For this review, take the finished solid that the model builds, in its own axes (mm). A direction names the side the tool comes from. Coordinates: 2 decimals unless noted, no trailing zeros.
1. Clearance check with flat-ended pins moving along their axes: P1, Ø7, axis at x = -2.5, y = 6, coming from the -Z side; P2, Ø2, axis at x = 0.5, y = 0, coming from the -Z side; P3, Ø3, axis at x = -0.5, y = -4.5, coming from the +Z side; P4, Ø5, axis at x = -2, z = 30, coming from the -Y side. State where each tip first meets the part, or that it passes through.
2. Mouldability with a two-part tool opening along X and no side actions: class faces 4 (the face through (-9, 3.5, 21)), 5 (the face through (0, 14, 18)) as pulls with the +X half, pulls with the -X half, needs draft (parallel to the pull), parting line crosses it, or undercut.
3. Take a section at A-A, the plane y = 5.5. Count the separate pieces of the cut face and the enclosed holes in it, then the cut area to 3 significant figures.
4. To check wall thickness, follow probe 1 along Z at (x, y) = (0, 9.5); probe 2 along X at (y, z) = (12.9, 25.5); probe 3 along Z at (x, y) = (-9, -6.25). State the ranges of each line that lie inside material, in increasing order.
5. Machinability: for faces 1 (the face through (0, -14, 1)), 2 (the face through (8.26, 0.39, 1.23)), 3 (the face through (0.46, 7.44, 5.81)), which of the approach directions +Z, -Z, +X, -X, +Y, -Y give a long, thin tool a straight path to every point of the face, cutting with its end or side? Answer none if there is none.
```python
from build123d import *

# Parameters (mm, degrees)
SKETCH1_W           = 33
SKETCH1_H           = 28
BOSS_EXTRUDE1_DEPTH = 46
CUT_EXTRUDE1_DEPTH  = 59.318093247
CUT_EXTRUDE2_START  = -3
CUT_EXTRUDE2_DEPTH  = 27
FILLET1_R           = 12.5
FILLET2_R           = 16.5
FILLET3_R           = 6
SKETCH4_W           = 13
SKETCH4_H           = 23
CUT_EXTRUDE3_DEPTH  = 9
SKETCH5_R           = 6.5
CUT_EXTRUDE4_DEPTH  = 56.592265809
SKETCH6_R           = 1
CUT_EXTRUDE6_DEPTH  = 8
SKETCH7_R           = 1.3
SKETCH7_R_2         = 2.5
CUT_EXTRUDE7_DEPTH  = 2.5


with BuildPart() as part:
    # Sketch1 → Boss-Extrude1 (new body)
    with BuildSketch(Plane.XY):
        Rectangle(SKETCH1_W, SKETCH1_H)
    extrude(amount=BOSS_EXTRUDE1_DEPTH)

    # Sketch2 → Cut-Extrude1 (cut, through all)
    with BuildSketch(Plane(origin=(16.5, 0, 0), x_dir=(0, 0, -1), z_dir=(1, 0, 0))):
        with BuildLine():
            Line((-46, 2), (-46, -14))
            Line((-46, -14), (-5, -14))
            add(Edge.make_bspline(
                [(-5, -14), (-24.736297584, -3.666123858), (-46, 2)],
                knots=[0, 0, 0, 1, 1, 1], degree=2))
        make_face()
    extrude(amount=-CUT_EXTRUDE1_DEPTH, mode=Mode.SUBTRACT)

    # Sketch3 → Cut-Extrude2 (cut)
    with BuildSketch(Plane(origin=(16.5, 0, 0), x_dir=(0, 0, -1), z_dir=(1, 0, 0)).offset(CUT_EXTRUDE2_START)):
        with BuildLine():
            Line((-5, -14), (-2.5, -14))
            Line((-2.5, -14), (-2.5, 3.5))
            Line((-2.5, 3.5), (-40.5, 3.5))
            Line((-40.5, 3.5), (-40.5, 0.448741524))
            add(Edge.make_bspline(
                [(-5, -14), (-22.171866916, -5.008853353), (-40.5, 0.448741524)],
                knots=[0, 0, 0, 1, 1, 1], degree=2))
        make_face()
    extrude(amount=-CUT_EXTRUDE2_DEPTH, mode=Mode.SUBTRACT)

    # Fillet1
    fillet1_edges = [part.edges().sort_by_distance(p)[0] for p in [
        (13.5, 1.974370762, 40.5),
        (-13.5, 1.974370762, 40.5),
    ]]
    fillet(fillet1_edges, radius=FILLET1_R)

    # Fillet2
    fillet2_edges = [part.edges().sort_by_distance(p)[0] for p in [
        (16.5, 8, 46),
        (-16.5, 8, 46),
    ]]
    fillet(fillet2_edges, radius=FILLET2_R - 0.0001)  # a hair under: the kernel refuses the full size

    # Fillet3
    fillet3_edges = [part.edges().sort_by_distance(p)[0] for p in [
        (-16.5, -14, 2.5),
        (16.5, -14, 2.5),
    ]]
    fillet(fillet3_edges, radius=FILLET3_R)

    # Sketch4 → Cut-Extrude3 (cut)
    with BuildSketch(Plane.XZ.offset(-3.5)):
        with Locations((0, 20.5)):
            Rectangle(SKETCH4_W, SKETCH4_H)
    extrude(amount=-CUT_EXTRUDE3_DEPTH, mode=Mode.SUBTRACT)

    # Sketch5 → Cut-Extrude4 (cut, through all)
    with BuildSketch(Plane.XZ.offset(-12.5)):
        with Locations((0, 25.5)):
            Circle(SKETCH5_R)
    extrude(amount=-CUT_EXTRUDE4_DEPTH, mode=Mode.SUBTRACT)

    # Sketch6 → Cut-Extrude6 (cut)
    with BuildSketch(Plane.XZ.offset(-3.5)):
        with Locations((0, 34.3)):
            Circle(SKETCH6_R)
        with Locations((0, 6.7)):
            Circle(SKETCH6_R)
    extrude(amount=-CUT_EXTRUDE6_DEPTH, mode=Mode.SUBTRACT)

    # Sketch7 → Cut-Extrude7 (cut)
    with BuildSketch(Plane(origin=(0, 0, 0), x_dir=(-1, 0, 0), z_dir=(0, 0, -1))):
        with Locations((-9.5, 0)):
            Circle(SKETCH7_R)
        with Locations((-5, 0)):
            Circle(SKETCH7_R_2)
        with Locations((-0.5, 0)):
            Circle(SKETCH7_R)
    extrude(amount=-CUT_EXTRUDE7_DEPTH, mode=Mode.SUBTRACT)


solid = part.part
```
Results list:
1. P1: stops at z = 0
1. P2: stops at z = 40.49
1. P3: stops at z = 2.5
1. P4: stops at y = 3.5
2. face 4: undercut
2. face 5: needs draft
3. separate pieces: 1
3. enclosed holes: 3
3. area: 1,100 mm2
4. probe 1: z = 0 to 5.7, 7.7 to 9, 32 to 33.3, 35.3 to 46
4. probe 2: x = -16.5 to -6.5, 6.5 to 16.5
4. probe 3: z = 0 to 2.5
5. face 1: +Z, -Z, +X, -X, -Y
5. face 2: -Z
5. face 3: -Y
